The model under review builds one solid part; all positions refer to its coordinate system, in mm. Coordinates: 2 decimals unless noted, no trailing zeros. Order: outer loops, then holes, each group sorted by start corner. A loop starts at its lowest first (then second) coordinate and runs counter-clockwise, first axis right, second up. Notation, with made-up numbers: (64, 13.5) -> (116, 13.5) arc R24 ccw to (116, 44.5) -> close; hole circle Ø1 at (75.25, 8). An arc over 180 degrees is marked (long way). Use one line per item in the form item = value.
from build123d import *

# Parameters (mm, degrees)
SKETCH1_W           = 100
SKETCH1_H           = 166
MAIN_BODY_DEPTH     = 3.5
SKETCH2_W           = 72
SKETCH2_H           = 40
PCBS_AND_SUCH_DEPTH = 5


with BuildPart() as part:
    # Sketch1 → MAIN BODY (new body)
    with BuildSketch(Plane(origin=(0, 0, 0), x_dir=(1, 0, 0), z_dir=(0, 1, 0))):
        Rectangle(SKETCH1_W, SKETCH1_H)
    extrude(amount=MAIN_BODY_DEPTH)

    # Sketch2 → PCBs AND SUCH (add)
    with BuildSketch(Plane.XZ):
        with Locations((-10, -63)):
            Rectangle(SKETCH2_W, SKETCH2_H)
    extrude(amount=PCBS_AND_SUCH_DEPTH)


solid = part.part
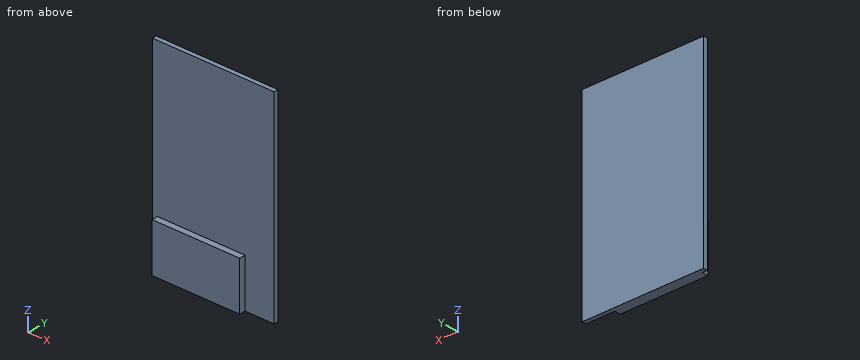
Item 1: We need section A-A (z = -65.5). Write out the cut boundary in (x, y), plus the area to 3 significant figures.
Results found:
outline = (-50, 0) -> (-46, 0) -> (-46, -5) -> (26, -5) -> (26, 0) -> (50, 0) -> (50, 3.5) -> (-50, 3.5) -> close
area = 710 mm²
Item 2: We need section D-D (x = 34.5). Write out the cut boundary in (y, z).
Results found:
outline = (0, -83) -> (3.5, -83) -> (3.5, 83) -> (0, 83) -> close
Item 3: We need section C-C (y = -3). Write out the cut boundary in (x, z), plus the area to 3 significant figures.
Results found:
outline = (-46, -83) -> (26, -83) -> (26, -43) -> (-46, -43) -> close
area = 2,880 mm²
Item 4: Clearance check with flat-ended pins moving along their axes: pin 1 (1 mm diameter, centred on x = -16.5, y = -2.5, fed in from +Z); pin 2 (4 mm diameter, centred on y = -3.5, z = 35, fed in from -X); pin 3 (12 mm diameter, centred on x = -7.5, z = 61, fed in from -Y). State where each tip first meets the part, or that it passes through.
Results found:
pin_1 = -43
pin_2 = through
pin_3 = 0
Item 5: We need section B-B (x = -39.5). Write out the cut boundary in (y, z).
Results found:
outline = (-5, -83) -> (3.5, -83) -> (3.5, 83) -> (0, 83) -> (0, -43) -> (-5, -43) -> close
Item 6: To check wall thickness, follow L1, parallel to Y at x = 38, z = 75; L2, parallel to Z at x = -16.5, y = -2.5; L3, parallel to X at y = -2.5, z = -63.5. State the ranges of each line that lie inside material, in increasing order. Write a range as from..to.
Results found:
L1 = 0..3.5
L2 = -83..-43
L3 = -46..26
